Check sheet for the modelled part. Datum: model origin and axes. Units: mm. A direction names the side the tool comes from. Coordinates: 2 decimals unless noted, no trailing zeros. Write each loop counter-clockwise with the first axis right and the second up, starting at its lowest first coordinate (ties: lowest second). Pieces come first, ordered by that corner, then holes. Notation, with made-up numbers: (57.5, 78.5) -> (74.5, 78.5) arc R28 ccw to (74.5, 114.5) -> close; hole circle Ø4 at (3.5, 74.5). An arc over 180 degrees is marked (long way). One line per item, written item: value. Start each with the question number.
1) Gauge pin test, flat end, axial feed: P1, Ø1.4, axis at y = 0, z = 3.5, coming from the -X side. Record the tip position at first contact, or that the pin passes through.
2) Draft check along Z on faces 5 (the cylindrical face through (2.41, 37.82, 3.28)), 6 (the cylindrical face through (-9.524, -0.07, 3.219)), 7 (the flat face through (-1, 10, 6.35)). Enter one of: +Z half, -Z half, draft (parallel to the pull), parting line (faces both ways), or undercut.
3) Sectioned sample at A-A on x = 0. Enter the section's corners in (y, z) (3 decimals).
4) Scan lines: line 1 along Y through (x, z) = (-3, 2.5) (3 decimals); line 2 along X through (y, z) = (20, 1); line 3 along Y through (x, z) = (45.5, 4.25) (3 decimals). Record each from-to range of solid material in increasing order. Write a range as [from, to].
5) Set-up check for faces 1 (the flat face through (0, -3.175, 3)), 2 (the flat face through (-42.862, 0, 3)), 3 (the cylindrical face through (2.41, -37.82, 3.28)), 4 (the cylindrical face through (49.301, -0.924, 0.946)): record each of +Z, -Z, +X, -X, +Y, -Y from which the full face is reachable in a straight line by a thin tool's end or side.
```python
from build123d import *

# Parameters (mm, degrees)
SKETCH1_W           = 111.125
SKETCH1_H           = 82.55
SKETCH1_R           = 4.7625
BOSS_EXTRUDE1_DEPTH = 6.35
SKETCH2_R           = 2.413
CUT_EXTRUDE1_DEPTH  = 12.7
SKETCH3_R           = 2.413
CUT_EXTRUDE2_DEPTH  = 12.7
CUT_EXTRUDE3_DEPTH  = 7.62


with BuildPart() as part:
    # Sketch1 → Boss-Extrude1 (new body)
    with BuildSketch(Plane.XY):
        Rectangle(SKETCH1_W, SKETCH1_H)
        with Locations((0, 30.1625)):
            Circle(SKETCH1_R, mode=Mode.SUBTRACT)
        with Locations(Location((0, -30.1625, 0), (0, 0, 180))):
            Circle(SKETCH1_R, mode=Mode.SUBTRACT)
    extrude(amount=BOSS_EXTRUDE1_DEPTH)

    # Sketch2 → Cut-Extrude1 (cut)
    with BuildSketch(Plane(origin=(55.5625, 0, 0), x_dir=(0, 0, -1), z_dir=(1, 0, 0))):
        with Locations((-3.175, 20.6375)):
            Circle(SKETCH2_R)
        with Locations((-3.175, 0)):
            Circle(SKETCH2_R)
        with Locations((-3.175, -20.6375)):
            Circle(SKETCH2_R)
    cut_extrude1 = extrude(amount=-CUT_EXTRUDE1_DEPTH, mode=Mode.SUBTRACT)

    # Mirror1: Cut-Extrude1 across plane
    add(cut_extrude1.mirror(Plane(origin=(0, 0, 0), x_dir=(0, 0, 1), z_dir=(1, 0, 0))), mode=Mode.SUBTRACT)

    # Sketch3 → Cut-Extrude2 (cut)
    with BuildSketch(Plane(origin=(0, 41.275, 0), x_dir=(1, 0, 0), z_dir=(0, 1, 0))):
        with Locations(Location((0, -3.175, 0), (0, 0, 180))):
            Circle(SKETCH3_R)
    cut_extrude2 = extrude(amount=-CUT_EXTRUDE2_DEPTH, mode=Mode.SUBTRACT)

    # Mirror2: Cut-Extrude2 across plane
    add(cut_extrude2.mirror(Plane.ZX), mode=Mode.SUBTRACT)

    # Sketch4 → Cut-Extrude3 (cut)
    with BuildSketch(Plane.XY.offset(6.35)):
        with BuildLine():
            Line((-6.35, 3.175), (6.35, 3.175))
            ThreePointArc((6.35, 3.175), (9.525, 0), (6.35, -3.175))
            Line((6.35, -3.175), (-6.35, -3.175))
            ThreePointArc((-6.35, -3.175), (-9.525, 0), (-6.35, 3.175))
        make_face()
    extrude(amount=-CUT_EXTRUDE3_DEPTH, mode=Mode.SUBTRACT)


solid = part.part
```
Answers:
1. P1: stops at x = -42.86
2. face 5: undercut
2. face 6: draft
2. face 7: +Z half
3. outline: (-41.275, 0) -> (-34.925, 0) -> (-34.925, 0.762) -> (-41.275, 0.762) -> close; (-41.275, 5.588) -> (-34.925, 5.588) -> (-34.925, 6.35) -> (-41.275, 6.35) -> close; (-25.4, 0) -> (-3.175, 0) -> (-3.175, 6.35) -> (-25.4, 6.35) -> close; (3.175, 0) -> (25.4, 0) -> (25.4, 6.35) -> (3.175, 6.35) -> close; (34.925, 0) -> (41.275, 0) -> (41.275, 0.762) -> (34.925, 0.762) -> close; (34.925, 5.588) -> (41.275, 5.588) -> (41.275, 6.35) -> (34.925, 6.35) -> close
4. line 1: y = [-41.275, -33.861], [-26.464, -3.175], [3.175, 26.464], [33.861, 41.275]
4. line 2: x = [-42.86, 42.86]
4. line 3: y = [-41.275, -22.798], [-18.477, -2.16], [2.16, 18.477], [22.798, 41.275]
5. face 1: +Z, -Z
5. face 2: -X
5. face 3: -Y
5. face 4: +X
